Design review of the part built by this model. Coordinates are the model's own, in mm. A direction names the side the tool comes from. Give positions to 0.01 mm unless a question says otherwise; leave off trailing zeros. Loops run counter-clockwise (first coordinate to the right, second up) from the corner with the lowest first, then second, coordinate; pieces in that order, holes last. Notation, with made-up numbers: M 72.5,32 L 87.5,32 A36 ccw 87.5,69 Z; hole C -10.5,42.5 d6. An arc over 180 degrees is marked long. Answer as CSV lines item,"result".
```python
from build123d import *

# Parameters (mm, degrees)
F2_R = 9
F3_R = 8.781681
F4_R = 17.563363
F5_R = 0.5


with BuildPart() as f1:
    # F0 (on Right) → F1 (revolve)
    with BuildSketch(Plane.YZ):
        Polygon((-63, 0), (0, 0), (0, 4.5), (-8, 4.5), (-18, 9), (-63, 9), align=None)
    revolve(axis=Axis((0, -31.5, 0), (0, 1, 0)))

    # F2
    f2_edges = [f1.edges().sort_by_distance(p)[0] for p in [
        (0, -63, -9),
    ]]
    fillet(f2_edges, radius=F2_R)

    # F3
    f3_edges = [f1.edges().sort_by_distance(p)[0] for p in [
        (0, -18, -9),
    ]]
    fillet(f3_edges, radius=F3_R)

    # F4
    f4_edges = [f1.edges().sort_by_distance(p)[0] for p in [
        (0, -12.140581, 6.363261),
        (0, -16.281162, -8.226521),
        (0, -8, -4.5),
    ]]
    fillet(f4_edges, radius=F4_R)

    # F5
    f5_edges = [f1.edges().sort_by_distance(p)[0] for p in [
        (0, 0, -4.5),
    ]]
    fillet(f5_edges, radius=F5_R)


solid = f1.part
```
1. We need section A-A, the plane y = -24. Write out the cut boundary in (x, z), plus the area to 3 significant figures.
Answer block:
outline,"C 0,0 d18"
area,"254 mm²"
2. To check wall thickness, follow L1, parallel to X at y = -25, z = -0.5; L2, parallel to Z at x = 0.25, y = -51; L3, parallel to Z at x = -4, y = -48. State the ranges of each line that lie inside material, in increasing order. Write a range as [from, to].
Answer block:
L1,"[-8.99, 8.99]"
L2,"[-9, 9]"
L3,"[-8.06, 8.06]"
3. For faces 1 (the cylindrical face through (2.703, -37.181, 8.584)), 2 (the cylindrical face through (1.352, -2.391, 4.292)), list the 3-axis set-ups (+Z, -Z, +X, -X, +Y, -Y) from which the entire face can be reached by the end or side of a thin tool; tool diameter is ignored.
Answer block:
face 1,"+Y, -Y"
face 2,"+Y"
4. For P1, Ø1, axis at y = -50, z = 3.5, coming from the +X side; P2, Ø1, axis at y = -38, z = -2, coming from the -X side; P3, Ø10, axis at x = -7, y = -41.5, coming from the +Z side; P4, Ø5, axis at x = 0, z = 4.5, coming from the +Y side, all flat-tipped, find the tip position at first contact; note any pin that passes through.
Answer block:
P1,"x = 8.49"
P2,"x = -8.87"
P3,"z = 8.77"
P4,"y = 0"
5. We need section B-B, the plane y = -55.5. Write out the cut boundary in (x, z), plus the area to 3 significant figures.
Answer block:
outline,"C 0,0 d17.75"
area,"247 mm²"
